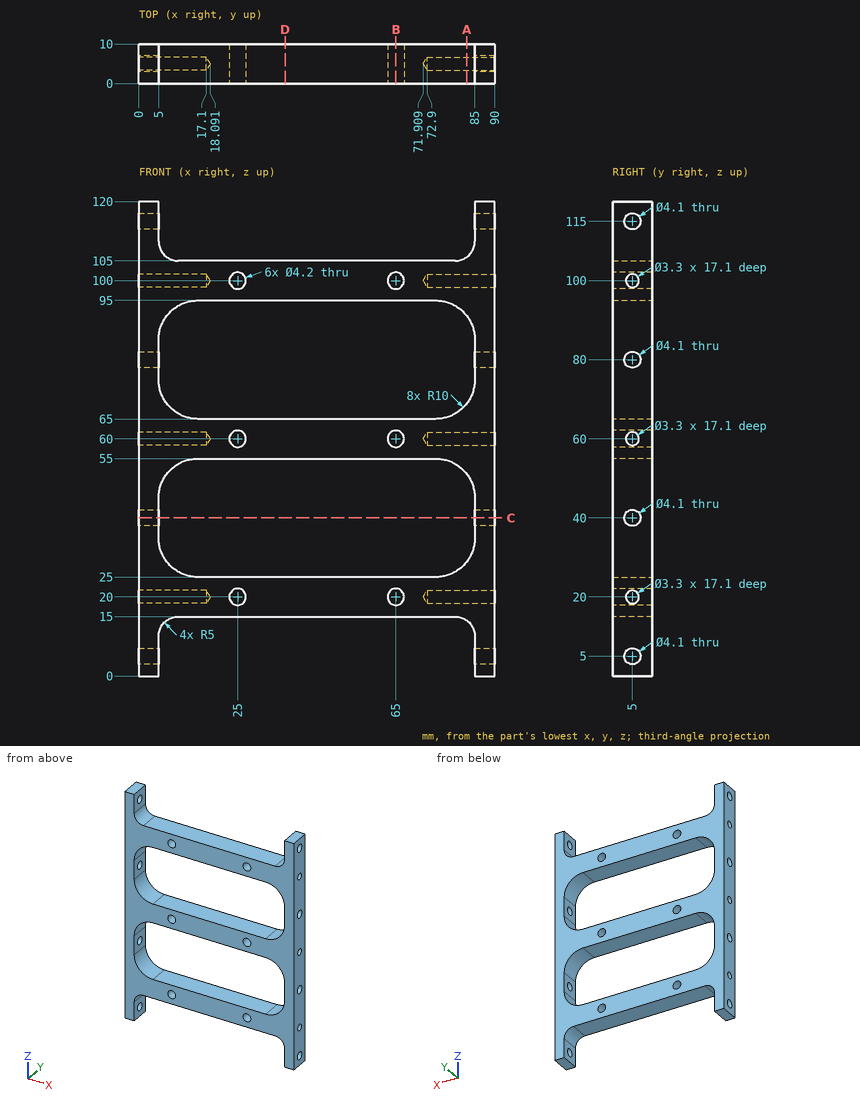
Verification items for this drawing (mm, ordinates from the low corner). Give positions to 0.01 mm unless a question says otherwise; leave off trailing zeros. Write each loop counter-clockwise with the first axis right and the second up, starting at its lowest first coordinate (ties: lowest second). Pieces come first, ordered by that corner, then holes. Notation, with made-up numbers: (79.25, -31) -> (100.25, -31) arc R23 ccw to (100.25, 6) -> close; hole circle Ø5 at (48.25, 76). An arc over 180 degrees is marked (long way). Use CSV: the item, a comma, the result in double quotes. Start each with the question number.
Q1. Cross-section at A-A on x = 83. Enter the section's corners in (y, z), and give its area (3 significant figures).
Q2. Scan lines: line 1 along Z through (x, y) = (32, 2.75); line 2 along Y through (x, z) = (2, 80); line 3 along X through (y, z) = (7.5, 100). Record each from-to range of solid material in increasing order.
Q3. Depth check by flat-ended pin: P1, Ø2.5, axis at y = 5, z = 115, coming from the +X side; P2, Ø5, axis at x = 45, y = 2.5, coming from the -Z side; P3, Ø5, axis at x = 17, y = 4, coming from the +Z side. Enter the tip coordinate at first touch or a pass-through.
Q4. Cross-section at C-C on z = 40. Enter the section's corners in (x, y).
Q5. Cross-section at B-B on x = 65. Enter the section's corners in (y, z).
Q6. Cross-section at D-D on x = 37. Enter the section's corners in (y, z).
Working result:
1,outline,"(0, 14) -> (10, 14) -> (10, 29) -> (0, 29) -> close; (0, 51) -> (10, 51) -> (10, 69) -> (0, 69) -> close; (0, 91) -> (10, 91) -> (10, 106) -> (0, 106) -> close; hole circle Ø3.3 at (5, 20); hole circle Ø3.3 at (5, 60); hole circle Ø3.3 at (5, 100)"
1,area,"454 mm^2"
2,line 1,"z = 15 to 25, 55 to 65, 95 to 105"
2,line 2,"y = 0 to 2.95, 7.05 to 10"
2,line 3,"x = 0 to 22.9, 27.1 to 62.9, 67.1 to 90"
3,P1,"passes through"
3,P2,"stops at z = 15"
3,P3,"stops at z = 105"
4,outline,"(0, 0) -> (5, 0) -> (5, 2.95) -> (0, 2.95) -> close; (0, 7.05) -> (5, 7.05) -> (5, 10) -> (0, 10) -> close; (85, 0) -> (90, 0) -> (90, 2.95) -> (85, 2.95) -> close; (85, 7.05) -> (90, 7.05) -> (90, 10) -> (85, 10) -> close"
5,outline,"(0, 15) -> (10, 15) -> (10, 17.9) -> (0, 17.9) -> close; (0, 22.1) -> (10, 22.1) -> (10, 25) -> (0, 25) -> close; (0, 55) -> (10, 55) -> (10, 57.9) -> (0, 57.9) -> close; (0, 62.1) -> (10, 62.1) -> (10, 65) -> (0, 65) -> close; (0, 95) -> (10, 95) -> (10, 97.9) -> (0, 97.9) -> close; (0, 102.1) -> (10, 102.1) -> (10, 105) -> (0, 105) -> close"
6,outline,"(0, 15) -> (10, 15) -> (10, 25) -> (0, 25) -> close; (0, 55) -> (10, 55) -> (10, 65) -> (0, 65) -> close; (0, 95) -> (10, 95) -> (10, 105) -> (0, 105) -> close"
